Read the model definition and answer for the solid it produces. Units are mm, in the model's axes. A direction names the side the tool comes from. Give positions to 0.01 mm unless a question says otherwise; leave off trailing zeros. Order: outer loops, then holes, each group sorted by start corner. A loop starts at its lowest first (then second) coordinate and runs counter-clockwise, first axis right, second up. Notation, with made-up numbers: (32, 81) - (67, 81) arc R20 cw to (67, 117) - close; hole circle Ø2 at (56, 58.25). An arc over 180 degrees is marked (long way). Use a Markdown table: item, result. Add a question column.
1. A cutting plane is placed at C-C on x = 1.5. Determine the outline of the cut face in (y, z), and give its area (3 significant figures).
2. A cutting plane is placed at B-B on z = 11. Determine the outline of the cut face in (x, y).
3. A cutting plane is placed at D-D on y = 6.5. Determine the outline of the cut face in (x, z), and give its area (3 significant figures).
4. Consider L1, parallel to X at y = 18.5, z = 8.75; L2, parallel to X at y = 12, z = 22. Determine where each line is inside the solid, lowest interval first.
5. A cutting plane is placed at A-A on y = 10.75. Determine the outline of the cut face in (x, z), and give its area (3 significant figures).
6. Which of the six approach directions +Z, -Z, +X, -X, +Y, -Y give full straight-line access (tool end or side, diameter ignored) to faces 5 (the flat face through (6.4, 6.3, 19)), 6 (the flat face through (-24, 21, 12.7)), 7 (the flat face through (-32, 6, 6)), 8 (the flat face through (-13, 19.05, 6)), 9 (the flat face through (0, 13, 13))?
7. For a pull along X with two mould halves and no side action, classify faces 1 (the flat face through (12.7, 13, 13)), 2 (the flat face through (-38.1, 16, 6)), 3 (the flat face through (6, 19, 25.4)), 4 (the flat face through (-25.4, 12, 5)) as released by +X, released by -X, zero draft, split by the parting line, or undercut.
8. Flat-ended cylindrical pins translate along their axes: P1, Ø3, axis at x = -13, y = 19.5, coming from the -Z side; P2, Ø4, axis at x = -20.5, y = 19, coming from the +Z side; P3, Ø14, axis at x = -13, z = 6.5, coming from the -Y side. Find the tip coordinate at first contact, or state that the pin passes through.
```python
from build123d import *

# Parameters (mm, degrees)
F0_W     = 25.4
F0_H     = 25.4
F1_DEPTH = 12.7
F2_W     = 6.35
F2_H     = 12.7
F3_DEPTH = 38.1
F4_W     = 12.7
F4_H     = 12.7
F5_DEPTH = 19.05
F7_DEPTH = 12.7
F9_DEPTH = 12.7


with BuildPart() as f1:
    # F0 (on Right) → F1 (new body)
    with BuildSketch(Plane.YZ):
        with Locations((12.7, 12.7)):
            Rectangle(F0_W, F0_H)
    extrude(amount=F1_DEPTH)

    # F2 (on Right) → F3 (join)
    with BuildSketch(Plane.YZ):
        with Locations((22.225, 6.35)):
            Rectangle(F2_W, F2_H)
    extrude(amount=-F3_DEPTH)

    # F4 (on face) → F5 (join)
    with BuildSketch(Plane.XZ.offset(-19.05)):
        with Locations((-31.75, 6.35)):
            Rectangle(F4_W, F4_H)
    extrude(amount=F5_DEPTH)

    # F6 (on face) → F7 (cut)
    with BuildSketch(Plane.YZ.offset(12.7)):
        Polygon((12.7, 25.4), (0, 25.4), (0, 12.7), align=None)
    extrude(amount=-F7_DEPTH, mode=Mode.SUBTRACT)

    # F8 (on face) → F9 (cut)
    with BuildSketch(Plane.YZ.offset(-25.4)):
        Polygon((12.7, 12.7), (0, 12.7), (0, 0), align=None)
    extrude(amount=-F9_DEPTH, mode=Mode.SUBTRACT)


solid = f1.part
```
Output values:
| question | item | result |
|---|---|---|
| 1 | outline | (0, 0) - (25.4, 0) - (25.4, 25.4) - (12.7, 25.4) - (0, 12.7) - close |
| 1 | area | 565 mm² |
| 2 | outline | (-38.1, 11) - (-25.4, 11) - (-25.4, 19.05) - (0, 19.05) - (0, 0) - (12.7, 0) - (12.7, 25.4) - (-38.1, 25.4) - close |
| 3 | outline | (-38.1, 0) - (-25.4, 0) - (-25.4, 6.5) - (-38.1, 6.5) - close; (0, 0) - (12.7, 0) - (12.7, 19.2) - (0, 19.2) - close |
| 3 | area | 326 mm² |
| 4 | L1 | -38.1 to -25.4, 0 to 12.7 |
| 4 | L2 | 0 to 12.7 |
| 5 | outline | (-38.1, 0) - (-25.4, 0) - (-25.4, 10.75) - (-38.1, 10.75) - close; (0, 0) - (12.7, 0) - (12.7, 23.45) - (0, 23.45) - close |
| 5 | area | 434 mm² |
| 6 | face 5 | +Z, +X, -X, -Y |
| 6 | face 6 | +Z, -X, +Y, -Y |
| 6 | face 7 | +Z, -X, -Y |
| 6 | face 8 | +Z, -Z, -Y |
| 6 | face 9 | +Z, -Y |
| 7 | face 1 | released by +X |
| 7 | face 2 | released by -X |
| 7 | face 3 | zero draft |
| 7 | face 4 | undercut |
| 8 | P1 | z = 0 |
| 8 | P2 | z = 12.7 |
| 8 | P3 | y = 19.05 |
